Geometry: see drawing. Coordinates: mm, zero at the bounding-box minimum. A direction names the side the tool comes from. Coordinates: 2 decimals unless noted, no trailing zeros. Loops run counter-clockwise (first coordinate to the right, second up) from the corner with the lowest first, then second, coordinate; pieces in that order, holes last. Notation, with made-up numbers: M 80,-13.5 L 122,-13.5 A27 ccw 122,2.5 Z; hole C -25.75,21 d2. An arc over 180 degrees is marked long. One line per question, with ' | ' between items. Start each with the question number.
1. Ray query, probe 1 along X at (y, z) = (0.9, 7); probe 2 along Z at (x, y) = (12, 2.25); probe 3 along Y at (x, z) = (8, 1.25). Return the intervals inside material, ascending.
2. Access query for the marked faces 4 and 5. Directions: +Z, -Z, +X, -X, +Y, -Y. A direction counts if a zero-diameter tool reaches every point of the face in a straight line with its end or side. Return the directions, or none.
3. Section query B-B, the plane x = 4. Output: boundary loops of the cut face in (y, z).
4. Pin query (flat end, axial travel): P1, Ø3, axis at x = 4, z = 7, coming from the +Y side; P2, Ø3, axis at x = 9, z = 6.5, coming from the -Y side; P3, Ø3, axis at x = 7.5, z = 9, coming from the +Y side; P4, Ø6, axis at x = 8, y = 28, coming from the +Z side. Return the tip coordinate at first contact, or that it passes through.
5. Section query D-D, the plane y = 5.5. Output: boundary loops of the cut face in (x, z), and give its area (3 significant figures).
6. Section query A-A, the plane z = 8.5. Output: boundary loops of the cut face in (x, y).
7. Section query C-C, the plane y = 28. Output: boundary loops of the cut face in (x, z), and give its area (3 significant figures).
8. Mould query, pull axis X, two halves, no side actions, for the marked faces 1, 2 and 3. Classes: pulls with the +X half, pulls with the -X half, needs draft (parallel to the pull), parting line crosses it, or undercut.
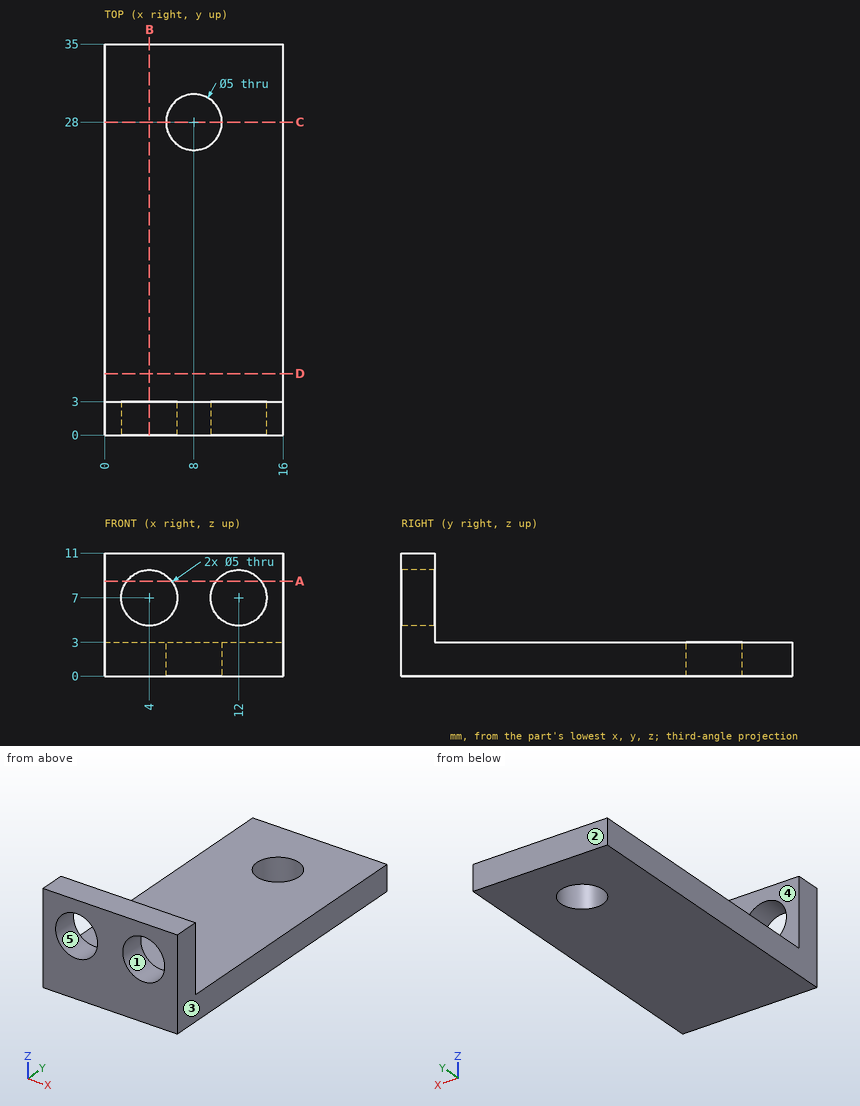
Taken from the geometry:
1) probe 1: 0 to 1.5, 6.5 to 9.5, 14.5 to 16 | probe 2: 0 to 4.5, 9.5 to 11 | probe 3: 0 to 25.5, 30.5 to 35
2) face 4: +Z, +X, -X, +Y | face 5: +Y, -Y
3) outline: M 0,0 L 35,0 L 35,3 L 3,3 L 3,4.5 L 0,4.5 Z; M 0,9.5 L 3,9.5 L 3,11 L 0,11 Z
4) P1: through | P2: y = 0 | P3: y = 3 | P4: z = 3
5) outline: M 0,0 L 16,0 L 16,3 L 0,3 Z | area: 48.0 mm^2
6) outline: M 0,0 L 2,0 L 2,3 L 0,3 Z; M 6,0 L 10,0 L 10,3 L 6,3 Z; M 14,0 L 16,0 L 16,3 L 14,3 Z
7) outline: M 0,0 L 5.5,0 L 5.5,3 L 0,3 Z; M 10.5,0 L 16,0 L 16,3 L 10.5,3 Z | area: 33.0 mm^2
8) face 1: undercut | face 2: needs draft | face 3: pulls with the +X half
